Could you check a few things on this model? Use its own coordinates, in mm. Give positions to 0.01 mm unless a question says otherwise; leave off trailing zeros. Loops run counter-clockwise (first coordinate to the right, second up) from the corner with the lowest first, then second, coordinate; pieces in that order, holes last. Notation, with made-up numbers: (39, -16.75) -> (58, -16.75) arc R21 ccw to (58, 18.25) -> close; hole circle Ø10 at (-28, 18). An arc over 180 degrees is marked (long way). Put each result on its own line as item: value.
Autodesk Inventor part; units mm, degrees
ref_plane "YZ Plane" through (0, 0, 0) normal (1, 0, 0) x (0, 1, 0)
ref_plane "XZ Plane" through (0, 0, 0) normal (0, 1, 0) x (-1, 0, 0)
ref_plane "XY Plane" through (0, 0, 0) normal (0, 0, 1) x (1, 0, 0)
sketch "Sketch1" plane through (0, 0, 0) normal (0, 1, 0) x (-1, 0, 0)
  line L0 (-230, 0) -> (-230, -280)
  line L1 (0, -280) -> (0, 0)
  line L2 (-115, 0) -> (-115, -280) construction
  line L3 (-230, -140) -> (0, -140) construction
  line L4 (0, -230) -> (-230, -230) construction
  line L5 (0, -28.043) -> (0, -96.333) construction
  line L6 (0, -69) -> (0, -31) construction
  line L7 (0, -50) -> (-230, -50) construction
  line L8 (0, -31) -> (-80, -31) construction
  line L9 (-80, -31) -> (-80, -69) construction
  line L10 (-80, -69) -> (0, -69) construction
  line L11 (0, -69) -> (0, -31)
  line L12 (-40, -50) -> (-40, -10.0475) construction
  line L13 (-40, -13.7025) -> (-29.2216, -13.7025)
  line L14 (-40, -13.7025) -> (-59.2216, -13.7025)
  line L15 (-29.2216, -13.7025) -> (-59.2216, -13.7025) construction
  line L16 (-29.2216, -11.7025) -> (-59.2216, -11.7025)
  line L17 (-59.2216, -15.7025) -> (-29.2216, -15.7025)
  arc A0 (-29.2216, -15.7025) -> (-29.2216, -11.7025) centre (-29.2216, -13.7025) ccw
  arc A1 (-59.2216, -11.7025) -> (-59.2216, -15.7025) centre (-59.2216, -13.7025) ccw
  line L18 (-40, -86.2975) -> (-29.2216, -86.2975)
  line L19 (-40, -86.2975) -> (-59.2216, -86.2975)
  line L20 (-29.2216, -86.2975) -> (-59.2216, -86.2975) construction
  line L21 (-29.2216, -88.2975) -> (-59.2216, -88.2975)
  line L22 (-59.2216, -84.2975) -> (-29.2216, -84.2975)
  arc A2 (-29.2216, -88.2975) -> (-29.2216, -84.2975) centre (-29.2216, -86.2975) ccw
  arc A3 (-59.2216, -84.2975) -> (-59.2216, -88.2975) centre (-59.2216, -86.2975) ccw
  line L23 (-230, -31) -> (-150, -31) construction
  line L24 (-150, -31) -> (-150, -69) construction
  line L25 (-150, -69) -> (-230, -69) construction
  line L26 (-190, -13.7025) -> (-200.7784, -13.7025)
  line L27 (-190, -13.7025) -> (-170.7784, -13.7025)
  line L28 (-200.7784, -13.7025) -> (-170.7784, -13.7025) construction
  line L29 (-200.7784, -11.7025) -> (-170.7784, -11.7025)
  line L30 (-170.7784, -15.7025) -> (-200.7784, -15.7025)
  arc A4 (-200.7784, -11.7025) -> (-200.7784, -15.7025) centre (-200.7784, -13.7025) ccw
  arc A5 (-170.7784, -15.7025) -> (-170.7784, -11.7025) centre (-170.7784, -13.7025) ccw
  arc A6 (-170.7784, -88.2975) -> (-170.7784, -84.2975) centre (-170.7784, -86.2975) ccw
  line L31 (-190, -86.2975) -> (-170.7784, -86.2975)
  line L32 (-170.7784, -84.2975) -> (-200.7784, -84.2975)
  line L33 (-190, -86.2975) -> (-200.7784, -86.2975)
  line L34 (-200.7784, -86.2975) -> (-170.7784, -86.2975) construction
  line L35 (-200.7784, -88.2975) -> (-170.7784, -88.2975)
  arc A7 (-200.7784, -84.2975) -> (-200.7784, -88.2975) centre (-200.7784, -86.2975) ccw
  line L36 (-115, -280) -> (-115, 0) construction
  line L37 (0, -230) -> (-230, -230) construction
  line L38 (0, -249) -> (-80, -249) construction
  line L39 (-80, -249) -> (-80, -211) construction
  line L40 (-80, -211) -> (0, -211) construction
  line L41 (-40, -230) -> (-40, -269.9525) construction
  line L42 (-40, -266.2975) -> (-29.2216, -266.2975)
  line L43 (-40, -266.2975) -> (-59.2216, -266.2975)
  line L44 (-29.2216, -266.2975) -> (-59.2216, -266.2975) construction
  line L45 (-29.2216, -268.2975) -> (-59.2216, -268.2975)
  line L46 (-59.2216, -264.2975) -> (-29.2216, -264.2975)
  arc A8 (-29.2216, -268.2975) -> (-29.2216, -264.2975) centre (-29.2216, -266.2975) ccw
  arc A9 (-59.2216, -264.2975) -> (-59.2216, -268.2975) centre (-59.2216, -266.2975) ccw
  arc A10 (-59.2216, -191.7025) -> (-59.2216, -195.7025) centre (-59.2216, -193.7025) ccw
  line L47 (-40, -193.7025) -> (-59.2216, -193.7025)
  line L48 (-59.2216, -195.7025) -> (-29.2216, -195.7025)
  line L49 (-40, -193.7025) -> (-29.2216, -193.7025)
  line L50 (-29.2216, -193.7025) -> (-59.2216, -193.7025) construction
  line L51 (-29.2216, -191.7025) -> (-59.2216, -191.7025)
  arc A11 (-29.2216, -195.7025) -> (-29.2216, -191.7025) centre (-29.2216, -193.7025) ccw
  line L52 (-150, -249) -> (-150, -211) construction
  line L53 (-170.7784, -264.2975) -> (-200.7784, -264.2975)
  line L54 (-190, -266.2975) -> (-200.7784, -266.2975)
  line L55 (-190, -266.2975) -> (-170.7784, -266.2975)
  arc A12 (-200.7784, -264.2975) -> (-200.7784, -268.2975) centre (-200.7784, -266.2975) ccw
  line L56 (-200.7784, -268.2975) -> (-170.7784, -268.2975)
  arc A13 (-170.7784, -268.2975) -> (-170.7784, -264.2975) centre (-170.7784, -266.2975) ccw
  line L57 (-200.7784, -266.2975) -> (-170.7784, -266.2975) construction
  line L58 (-170.7784, -195.7025) -> (-200.7784, -195.7025)
  line L59 (-190, -193.7025) -> (-200.7784, -193.7025)
  arc A14 (-200.7784, -191.7025) -> (-200.7784, -195.7025) centre (-200.7784, -193.7025) ccw
  line L60 (-200.7784, -193.7025) -> (-170.7784, -193.7025) construction
  line L61 (-200.7784, -191.7025) -> (-170.7784, -191.7025)
  line L62 (-190, -193.7025) -> (-170.7784, -193.7025)
  arc A15 (-170.7784, -195.7025) -> (-170.7784, -191.7025) centre (-170.7784, -193.7025) ccw
  line L63 (-150, -211) -> (-230, -211) construction
  line L64 (-230, -249) -> (-150, -249) construction
  line L65 (-192.5048, 9.5806) -> (-30, 9.5806)
  line L66 (-192.5048, -289.5806) -> (-30, -289.5806)
  line L67 (-80, -5) -> (-150, -5)
  line L68 (-150, -5) -> (-150, 5)
  line L69 (-150, 5) -> (-80, 5)
  line L70 (-80, 5) -> (-80, -5)
  line L71 (-80, -275) -> (-150, -275)
  line L72 (-150, -275) -> (-150, -285)
  line L73 (-150, -285) -> (-80, -285)
  line L74 (-80, -285) -> (-80, -275)
  line L75 (0, 0) -> (0, 9.5806)
  line L76 (0, 9.5806) -> (-30, 9.5806)
  line L77 (-192.5048, 9.5806) -> (-230, 9.5806)
  line L78 (-230, 9.5806) -> (-230, 0)
  line L79 (0, -280) -> (0, -289.5806)
  line L80 (0, -289.5806) -> (-30, -289.5806)
  line L81 (-192.5048, -289.5806) -> (-230, -289.5806)
  line L82 (-230, -289.5806) -> (-230, -280)
  point P0 (-40, -31)
  point P1 (-44.2216, -13.7025)
  point P2 (-44.2216, -86.2975)
  point P3 (-190, -50)
  point P4 (-190, -31)
  point P5 (-185.7784, -13.7025)
  point P6 (-185.7784, -86.2975)
  point P7 (-40, -249)
  point P8 (-44.2216, -266.2975)
  point P9 (-44.2216, -193.7025)
  point P10 (-190, -230)
  point P11 (-190, -249)
  point P12 (-185.7784, -193.7025)
  point P13 (-185.7784, -266.2975)
  point P14 (-115, -5)
  point P15 (-44.2216, -86.2975)
  point P16 (-44.2216, -193.7025)
  point P17 (-115, -280)
  point P18 (-115, -280)
  point P19 (-115, -275)
  dimension "d0" = 230
  dimension "d15" = 80
  dimension "d25" = 4
  dimension "d33" = 72.595
  dimension "d34" = 30
  dimension "d35" = 107.405
  dimension "d36" = 280
extrude "Extrusion1" add sketch "Sketch1" along normal blind 10 contours L78 L77 L65 L76 L75 L1 L79 L80 L66 L81 L82 L0 | A0 L17 A1 L16 | L21 A3 L22 A2 | L29 A5 L30 A4 | L35 A7 L32 A6 | L45 A9 L46 A8 | L51 A11 L48 A10 | A13 L56 A12 L53 | L58 A14 L61 A15 | L67 L68 L69 L70 | L74 L73 L72 L71
extrude "Extrusion2" cut sketch "Sketch1" along normal through all contours A0 L17 A1 L16 | L21 A3 L22 A2 | L29 A5 L30 A4 | L35 A7 L32 A6 | L45 A9 L46 A8 | L51 A11 L48 A10 | A13 L56 A12 L53 | L58 A14 L61 A15
extrude "Extrusion4" add sketch "Sketch1" along normal blind 10 contours L78 L77 L65 L76 L75 L1 L79 L80 L66 L81 L82 L0 | A0 L17 A1 L16 | L21 A3 L22 A2 | L29 A5 L30 A4 | L35 A7 L32 A6 | L45 A9 L46 A8 | L51 A11 L48 A10 | A13 L56 A12 L53 | L58 A14 L61 A15 | L67 L68 L69 L70 | L74 L73 L72 L71
extrude "Extrusion5" cut sketch "Sketch1" along normal blind 10 contours L67 L68 L69 L70 | L74 L73 L72 L71
extrude "Extrusion6" cut sketch "Sketch1" along normal blind 10 contours L29 A5 L30 A4
extrude "Extrusion7" cut sketch "Sketch1" along normal blind 10 contours A0 L17 A1 L16 | L21 A3 L22 A2 | L35 A7 L32 A6 | L45 A9 L46 A8 | L51 A11 L48 A10 | A13 L56 A12 L53 | L58 A14 L61 A15
properties part number "base"
1. If we section it at C-C (y = 1.5): Count the separate pieces of the cut face and the enclosed holes in it, then the cut area to 3 significant figures.
Recorded:
separate pieces: 1
enclosed holes: 10
area: 66,300 mm^2
2. If we section it at B-B (x = 32.5): List the corners of the cut face in (y, z) for me.
Recorded:
outline: (0, -289.58) -> (10, -289.58) -> (10, -268.3) -> (0, -268.3) -> close; (0, -264.3) -> (10, -264.3) -> (10, -195.7) -> (0, -195.7) -> close; (0, -191.7) -> (10, -191.7) -> (10, -88.3) -> (0, -88.3) -> close; (0, -84.3) -> (10, -84.3) -> (10, -15.7) -> (0, -15.7) -> close; (0, -11.7) -> (10, -11.7) -> (10, 9.58) -> (0, 9.58) -> close
3. I need wall thicknesses on line 1 (Z direction, x = 39, y = 6.75); line 2 (Z direction, x = 93, y = 6.75); line 3 (Z direction, x = 170, y = 6). Which ranges of each line are inside material? Lowest first, please.
Recorded:
line 1: z = -289.58 to -268.3, -264.3 to -195.7, -191.7 to -88.3, -84.3 to -15.7, -11.7 to 9.58
line 2: z = -289.58 to -285, -275 to -5, 5 to 9.58
line 3: z = -289.58 to -268.14, -264.46 to -195.54, -191.86 to -88.14, -84.46 to -15.54, -11.86 to 9.58
4. Thinking about a two-plate mould opening in Z: for faces 1 (the face through (44, 5, -88.298)), 2 (the face through (113, 5, -289.581)), 3 (the face through (230, 5, -138)), which applies, pulls with the +Z half, pulls with the -Z half, needs draft (parallel to the pull), parting line crosses it, or undercut?
Recorded:
face 1: undercut
face 2: pulls with the -Z half
face 3: needs draft
5. If we section it at A-A (x = 146.5): List the corners of the cut face in (y, z) for me.
Recorded:
outline: (0, -289.58) -> (10, -289.58) -> (10, -285) -> (0, -285) -> close; (0, -275) -> (10, -275) -> (10, -5) -> (0, -5) -> close; (0, 5) -> (10, 5) -> (10, 9.58) -> (0, 9.58) -> close
6. I'm going to push a flat-ended pin straight in: pin 1 (1.5 mm diameter, centred on y = 7.5, z = -234.5, fed in from -X). Where does the tip first touch, or does it pass through?
Recorded:
pin 1: stops at x = 0
